```python
from build123d import *

# Parameters (mm, degrees)
SKETCH_1_W          = 71
SKETCH_1_H          = 100
EXTRUDE_1_DEPTH     = 3
SKETCH_2_W          = 3
SKETCH_2_H          = 100
EXTRUDE_2_DEPTH     = 30
CUT_EXTRUDE_1_REACH = 94.898
SKETCH_3_R          = 4


with BuildPart() as part:
    # 草图1 → 凸台-拉伸1 (new body)
    with BuildSketch(Plane(origin=(0, 0, 0), x_dir=(1, 0, 0), z_dir=(0, 1, 0))):
        Rectangle(SKETCH_1_W, SKETCH_1_H)
    extrude(amount=EXTRUDE_1_DEPTH)

    # 草图2 → 凸台-拉伸2 (add)
    with BuildSketch(Plane(origin=(0, 3, 0), x_dir=(1, 0, 0), z_dir=(0, 1, 0))):
        with Locations((-34, 0)):
            Rectangle(SKETCH_2_W, SKETCH_2_H)
        with Locations((34, 0)):
            Rectangle(SKETCH_2_W, SKETCH_2_H)
    extrude(amount=EXTRUDE_2_DEPTH)

    # 切除-拉伸1: up to this face of the body (flat: up to its plane)
    cut_extrude_1_end = Plane(part.part.faces().sort_by_distance((-35.5, 16.5, 0))[0])
    # 草图3 → 切除-拉伸1 (cut, up to the picked face)
    with BuildSketch(Plane(origin=(35.5, 0, 0), x_dir=(0, 0, -1), z_dir=(1, 0, 0)), mode=Mode.PRIVATE) as cut_extrude_1_sk1:
        with Locations((42.5, 16.5)):
            Circle(SKETCH_3_R)
    cut_extrude_1_tool1 = split(extrude(cut_extrude_1_sk1.sketch, amount=-CUT_EXTRUDE_1_REACH, mode=Mode.PRIVATE), bisect_by=cut_extrude_1_end, keep=Keep.BOTH, mode=Mode.PRIVATE)
    # 草图3 → 切除-拉伸1 (cut, up to the picked face)
    with BuildSketch(Plane(origin=(35.5, 0, 0), x_dir=(0, 0, -1), z_dir=(1, 0, 0)), mode=Mode.PRIVATE) as cut_extrude_1_sk2:
        with BuildLine():
            Line((-42.5, 12.5), (17.5, 12.5))
            ThreePointArc((17.5, 12.5), (21.5, 16.5), (17.5, 20.5))
            Line((17.5, 20.5), (-42.5, 20.5))
            ThreePointArc((-42.5, 20.5), (-46.5, 16.5), (-42.5, 12.5))
        make_face()
    cut_extrude_1_tool2 = split(extrude(cut_extrude_1_sk2.sketch, amount=-CUT_EXTRUDE_1_REACH, mode=Mode.PRIVATE), bisect_by=cut_extrude_1_end, keep=Keep.BOTH, mode=Mode.PRIVATE)
    add(cut_extrude_1_tool1.solids().sort_by(Axis((35.5, 16.5, -42.5), (-1, 0, 0)))[0], mode=Mode.SUBTRACT)
    add(cut_extrude_1_tool2.solids().sort_by(Axis((35.5, 16.5, 12.5), (-1, 0, 0)))[0], mode=Mode.SUBTRACT)


solid = part.part
```
The listing builds one solid part. Answer for the finished solid, in the listing's coordinates (mm). A direction names the side the tool comes from. Give positions to 0.01 mm unless a question says otherwise; leave off trailing zeros. Order: outer loops, then holes, each group sorted by start corner. A loop starts at its lowest first (then second) coordinate and runs counter-clockwise, first axis right, second up. Notation, with made-up numbers: (75.5, 6) -> (97.5, 6) arc R13 cw to (97.5, 19) -> close; hole circle Ø2 at (24, -16.75). An arc over 180 degrees is marked (long way). Answer as CSV lines item,"result". Start each with the question number.
Q1. A cutting plane is placed at B-B (y = 16.5). Determine the outline of the cut face in (x, z), then the cut area to 3 significant figures.
Q2. A cutting plane is placed at D-D (x = 7.5). Determine the outline of the cut face in (y, z), then the cut area to 3 significant figures.
Q3. A cutting plane is placed at C-C (z = -25). Determine the outline of the cut face in (x, y).
Q4. A cutting plane is placed at A-A (z = -42.5). Determine the outline of the cut face in (x, y).
Q5. Find the intervals of material crossed by L1, parallel to Y at x = -34.3, z = -42.5; L2, parallel to X at y = 28.5, z = -20.5; L3, parallel to Z at x = -34, y = 16, in increasing order.
Q6. Which of the six approach directions +Z, -Z, +X, -X, +Y, -Y give full straight-line access (tool end or side, diameter ignored) to faces 1 (the flat face through (0, 0, -1)), 2 (the cylindrical face through (34, 16.4, -21.5)), 3 (the flat face through (0, 3, -1))?
Q7. Given pin 1 (6 mm diameter, centred on x = 19, z = -6, fed in from +Y), flat-ended and moving along its own axis, determine where the tip first touches the part or whether it passes through.
Q8. Determine the mould class of faces 4 (the flat face through (0, 2, 50)), 5 (the flat face through (34, 12.5, 13)), 6 (the flat face through (-34, 33, -1)) for opening direction Z: pulls with the +Z half, pulls with the -Z half, needs draft (parallel to the pull), parting line crosses it, or undercut.
Results found:
1,outline,"(-35.5, -50) -> (-32.5, -50) -> (-32.5, -46.5) -> (-35.5, -46.5) -> close; (-35.5, -38.5) -> (-32.5, -38.5) -> (-32.5, -21.5) -> (-35.5, -21.5) -> close; (-35.5, 46.5) -> (-32.5, 46.5) -> (-32.5, 50) -> (-35.5, 50) -> close; (32.5, -50) -> (35.5, -50) -> (35.5, -46.5) -> (32.5, -46.5) -> close; (32.5, -38.5) -> (35.5, -38.5) -> (35.5, -21.5) -> (32.5, -21.5) -> close; (32.5, 46.5) -> (35.5, 46.5) -> (35.5, 50) -> (32.5, 50) -> close"
1,area,"144 mm2"
2,outline,"(0, -50) -> (3, -50) -> (3, 50) -> (0, 50) -> close"
2,area,"300 mm2"
3,outline,"(-35.5, 0) -> (35.5, 0) -> (35.5, 33) -> (32.5, 33) -> (32.5, 3) -> (-32.5, 3) -> (-32.5, 33) -> (-35.5, 33) -> close"
4,outline,"(-35.5, 0) -> (35.5, 0) -> (35.5, 12.5) -> (32.5, 12.5) -> (32.5, 3) -> (-32.5, 3) -> (-32.5, 12.5) -> (-35.5, 12.5) -> close; (-35.5, 20.5) -> (-32.5, 20.5) -> (-32.5, 33) -> (-35.5, 33) -> close; (32.5, 20.5) -> (35.5, 20.5) -> (35.5, 33) -> (32.5, 33) -> close"
5,L1,"0 to 12.5, 20.5 to 33"
5,L2,"-35.5 to -32.5, 32.5 to 35.5"
5,L3,"-50 to -46.47, -38.53 to -21.47, 46.47 to 50"
6,face 1,"+Z, -Z, +X, -X, -Y"
6,face 2,"+X, -X"
6,face 3,"+Z, -Z, +Y"
7,pin 1,"y = 3"
8,face 4,"pulls with the +Z half"
8,face 5,"undercut"
8,face 6,"needs draft"
